Autodesk Inventor part; units mm, degrees
ref_plane "YZ Plane" through (0, 0, 0) normal (1, 0, 0) x (0, 1, 0)
ref_plane "XZ Plane" through (0, 0, 0) normal (0, 1, 0) x (-1, 0, 0)
ref_plane "XY Plane" through (0, 0, 0) normal (0, 0, 1) x (1, 0, 0)
sketch "Sketch1" plane through (0, 0, 0) normal (0, 1, 0) x (-1, 0, 0)
  line L0 (0, 0) -> (3.0988, 0)
  line L1 (3.0988, 0) -> (3.0988, -47.498)
  line L2 (3.0988, -47.498) -> (0, -47.498)
  line L3 (0, -47.498) -> (0, 0)
  line L4 (3.0988, 0) -> (0, 0)
  line L5 (0, 0) -> (0, -49.53)
  line L6 (0, -49.53) -> (3.0988, -49.53)
  line L7 (3.0988, -49.53) -> (3.0988, 0)
  dimension "d0" = 3.0988
  dimension "d1" = 47.498
  dimension "d2" = 49.53
revolve "top base" add sketch "Sketch1" angle 360 about axis through (-3.0988, 0, 0) along (1, 0, 0)
sketch "outer wall" plane through (0, 0, 0) normal (1, 0, 0) x (0, 0, -1)
  circle A0 centre (0, 0) radius 48.26
  circle A1 centre (0, 0) radius 49.53
  dimension "d4" = 96.52
  dimension "d7" = 99.06
extrude "top outer wall" add sketch "outer wall" along normal blind 17.78
sketch "top circles" plane through (0, 0, 0) normal (1, 0, 0) x (0, 0, -1)
  line L0 (27.4022, -6.3354) -> (27.4022, 6.3646) construction
  circle A0 centre (34.8952, 0.0146) radius 2.794
  circle A1 centre (19.9092, 0.0146) radius 2.794
  line L1 (22.7032, 0.0146) -> (32.1012, 0.0146) construction
  line L2 (14.7022, -6.3354) -> (40.1022, -6.3354) construction
  line L3 (40.1022, -6.3354) -> (40.1022, 6.3646) construction
  line L4 (40.1022, 6.3646) -> (14.7022, 6.3646) construction
  line L5 (14.7022, 6.3646) -> (14.7022, -6.3354) construction
  line L6 (14.7022, -6.3354) -> (40.1022, 6.3646) construction
  line L7 (40.1022, -6.3354) -> (14.7022, 6.3646) construction
  line L8 (40.065, -6.3646) -> (-40.065, -6.3646)
  line L9 (-40.065, -6.3646) -> (-40.065, 6.3646)
  line L10 (-40.065, 6.3646) -> (40.065, 6.3646)
  line L11 (40.065, 6.3646) -> (40.065, -6.3646)
  line L12 (40.065, -6.3646) -> (-40.065, 6.3646) construction
  line L13 (-40.065, -6.3646) -> (40.065, 6.3646) construction
  circle A2 centre (0, 0) radius 48.26
  point P0 (27.4022, 0.0146)
  dimension "d30" = 9.398
  dimension "d31" = 8.001
  dimension "d32" = 8.001
  dimension "d33" = 80.13
extrude "Top holes" cut sketch "top circles" against normal blind 25.4 contours A0 | A1
properties part number "Top Sensor Base v1.2"
For this review, take the finished solid that the model builds, in its own axes (mm). A direction names the side the tool comes from. Round coordinates to 2 decimals unless told otherwise and drop trailing zeros. Loops run counter-clockwise (first coordinate to the right, second up) from the corner with the lowest first, then second, coordinate; pieces in that order, holes last.
(1) We need section C-C (y = -15). Give the boundary of the cut face in (x, z), plus the area to 3 significant figures.
Returned:
outline: (-3.1, -47.2) - (17.78, -47.2) - (17.78, -45.87) - (0, -45.87) - (0, 45.87) - (17.78, 45.87) - (17.78, 47.2) - (-3.1, 47.2) - close
area: 340 mm2
(2) We need section A-A (z = -9). Give the boundary of the cut face in (x, y), plus the area to 3 significant figures.
Returned:
outline: (-3.1, -48.71) - (17.78, -48.71) - (17.78, -47.41) - (0, -47.41) - (0, 47.41) - (17.78, 47.41) - (17.78, 48.71) - (-3.1, 48.71) - close
area: 348 mm2
(3) Clearance check with flat-ended pins moving along their axes: P1, Ø10, axis at x = 2.5, z = 16, coming from the +Y side; P2, Ø1.5, axis at x = 3.5, z = 30, coming from the +Y side; P3, Ø9, axis at y = 0.01, z = -34.9, coming from the -X side; P4, Ø4, axis at x = 10.5, z = 9, coming from the -Y side. State where each tip first meets the part, or that it passes through.
Returned:
P1: stops at y = 48.29
P2: stops at y = 39.97
P3: stops at x = -3.1
P4: stops at y = -49.03
(4) Wall thickness on line 1 along Y through (x, z) = (2.5, 0); line 2 along X through (y, z) = (-28, 3); line 3 along Y through (x, z) = (1.5, 11.5): over which ranges is each line inside the solid? List them lowest first.
Returned:
line 1: y = -49.53 to -48.26, 48.26 to 49.53
line 2: x = -3.1 to 0
line 3: y = -48.18 to -46.87, 46.87 to 48.18
(5) Tool access review of faces 4 (the cylindrical face through (8.77, -14.5, -46.03)), 5 (the cylindrical face through (-1.53, -1.69, -32.68)): name each direction out of +Z, -Z, +X, -X, +Y, -Y from which nothing blocks a thin tool from reaching the whole face with its end or side.
Returned:
face 4: +X
face 5: +X, -X
(6) We need section B-B (x = 9.5). Give the boundary of the cut face in (y, z).
Returned:
outline: circle Ø99.06 at (0, 0); hole circle Ø96.52 at (0, 0)
(7) Mouldability with a two-part tool opening along Y and no side actions: class faces 1 (the cylindrical face through (7.19, -14.88, -47.24)), 2 (the flat face through (0, 1, 1)), 3 (the flat face through (17.78, -47.5, -10.8)) as released by +Y, released by -Y, zero draft, split by the parting line, or undercut.
Returned:
face 1: split by the parting line
face 2: undercut
face 3: zero draft
